Autodesk Inventor part; units mm, degrees
ref_plane "YZ Plane" through (0, 0, 0) normal (1, 0, 0) x (0, 1, 0)
ref_plane "XZ Plane" through (0, 0, 0) normal (0, 1, 0) x (-1, 0, 0)
ref_plane "XY Plane" through (0, 0, 0) normal (0, 0, 1) x (1, 0, 0)
sketch "Boceto1" plane through (0, 0, 0) normal (0, 0, 1) x (-1, 0, 0)
  line L0 (-40.5654, -5.9984) -> (-40.5654, 6.2017)
  line L1 (-40.5654, 6.2017) -> (-40.4637, 6.2017)
  line L2 (-40.4637, 6.2017) -> (-37.4137, 6.2017)
  line L3 (-37.4137, 6.2017) -> (-37.312, 6.2017)
  line L4 (-37.312, 6.2017) -> (-37.312, -5.9984)
  line L5 (-37.312, -5.9984) -> (-37.4137, -5.9984)
  line L6 (-37.4137, -5.9984) -> (-40.4637, -5.9984)
  line L7 (-40.4637, -5.9984) -> (-40.5654, -5.9984)
  line L8 (35.787, -5.9984) -> (35.6854, -5.9984)
  line L9 (35.6854, -5.9984) -> (32.6353, -5.9984)
  line L10 (32.6353, -5.9984) -> (32.5337, -5.9984)
  line L11 (32.5337, -5.9984) -> (32.5337, 6.2017)
  line L12 (32.5337, 6.2017) -> (32.6353, 6.2017)
  line L13 (32.6353, 6.2017) -> (35.6854, 6.2017)
  line L14 (35.6854, 6.2017) -> (35.787, 6.2017)
  line L15 (35.787, 6.2017) -> (35.787, -5.9984)
  line L16 (35.6854, 36.4987) -> (35.787, 36.4987)
  line L17 (35.787, 36.4987) -> (35.787, 24.2986)
  line L18 (35.787, 24.2986) -> (35.6854, 24.2986)
  line L19 (35.6854, 24.2986) -> (32.6353, 24.2986)
  line L20 (32.6353, 24.2986) -> (32.5337, 24.2986)
  line L21 (32.5337, 24.2986) -> (32.5337, 36.4987)
  line L22 (32.5337, 36.4987) -> (32.6353, 36.4987)
  line L23 (32.6353, 36.4987) -> (35.6854, 36.4987)
  line L24 (-26.0015, -48.4955) -> (-26.0015, -48.3938)
  line L25 (-26.0015, -48.3938) -> (-26.0015, -45.3438)
  line L26 (-26.0015, -45.3438) -> (-26.0015, -45.2421)
  line L27 (-26.0015, -45.2421) -> (-13.8014, -45.2421)
  line L28 (-13.8014, -45.2421) -> (-13.8014, -45.3438)
  line L29 (-13.8014, -45.3438) -> (-13.8014, -48.3938)
  line L30 (-13.8014, -48.3938) -> (-13.8014, -48.4955)
  line L31 (-13.8014, -48.4955) -> (-26.0015, -48.4955)
  line L32 (9.023, 45.4455) -> (9.023, 45.5471)
  line L33 (9.023, 45.5471) -> (9.023, 48.5971)
  line L34 (9.023, 48.5971) -> (9.023, 48.6988)
  line L35 (9.023, 48.6988) -> (21.2231, 48.6988)
  line L36 (21.2231, 48.6988) -> (21.2231, 48.5971)
  line L37 (21.2231, 48.5971) -> (21.2231, 45.5471)
  line L38 (21.2231, 45.5471) -> (21.2231, 45.4455)
  line L39 (21.2231, 45.4455) -> (9.023, 45.4455)
  line L40 (-26.0015, 45.4455) -> (-26.0015, 45.5471)
  line L41 (-26.0015, 45.5471) -> (-26.0015, 48.5971)
  line L42 (-26.0015, 48.5971) -> (-26.0015, 48.6988)
  line L43 (-26.0015, 48.6988) -> (-13.8014, 48.6988)
  line L44 (-13.8014, 48.6988) -> (-13.8014, 48.5971)
  line L45 (-13.8014, 48.5971) -> (-13.8014, 45.5471)
  line L46 (-13.8014, 45.5471) -> (-13.8014, 45.4455)
  line L47 (-13.8014, 45.4455) -> (-26.0015, 45.4455)
  line L48 (32.6353, -24.0952) -> (35.6854, -24.0952)
  line L49 (35.6854, -24.0952) -> (35.787, -24.0952)
  line L50 (35.787, -24.0952) -> (35.787, -36.2954)
  line L51 (35.787, -36.2954) -> (35.6854, -36.2954)
  line L52 (35.6854, -36.2954) -> (32.6353, -36.2954)
  line L53 (32.6353, -36.2954) -> (32.5337, -36.2954)
  line L54 (32.5337, -36.2954) -> (32.5337, -24.0952)
  line L55 (32.5337, -24.0952) -> (32.6353, -24.0952)
  line L56 (9.023, -48.4955) -> (9.023, -48.3938)
  line L57 (9.023, -48.3938) -> (9.023, -45.3438)
  line L58 (9.023, -45.3438) -> (9.023, -45.2421)
  line L59 (9.023, -45.2421) -> (21.2231, -45.2421)
  line L60 (21.2231, -45.2421) -> (21.2231, -45.3438)
  line L61 (21.2231, -45.3438) -> (21.2231, -48.3938)
  line L62 (21.2231, -48.3938) -> (21.2231, -48.4955)
  line L63 (21.2231, -48.4955) -> (9.023, -48.4955)
  line L64 (-37.4137, -36.2954) -> (-40.4637, -36.2954)
  line L65 (-40.4637, -36.2954) -> (-40.5654, -36.2954)
  line L66 (-40.5654, -36.2954) -> (-40.5654, -24.0952)
  line L67 (-40.5654, -24.0952) -> (-40.4637, -24.0952)
  line L68 (-40.4637, -24.0952) -> (-37.4137, -24.0952)
  line L69 (-37.4137, -24.0952) -> (-37.312, -24.0952)
  line L70 (-37.312, -24.0952) -> (-37.312, -36.2954)
  line L71 (-37.312, -36.2954) -> (-37.4137, -36.2954)
  line L72 (-37.312, 36.4987) -> (-37.312, 24.2986)
  line L73 (-37.312, 24.2986) -> (-37.4137, 24.2986)
  line L74 (-37.4137, 24.2986) -> (-40.4637, 24.2986)
  line L75 (-40.4637, 24.2986) -> (-40.5654, 24.2986)
  line L76 (-40.5654, 24.2986) -> (-40.5654, 36.4987)
  line L77 (-40.5654, 36.4987) -> (-40.4637, 36.4987)
  line L78 (-40.4637, 36.4987) -> (-37.4137, 36.4987)
  line L79 (-37.4137, 36.4987) -> (-37.312, 36.4987)
  line L80 (-3.05, -23.6886) -> (3.05, -23.6886)
  line L81 (3.05, -23.6886) -> (3.05, -30.8053)
  line L82 (3.05, -30.8053) -> (-3.05, -30.8053)
  line L83 (-3.05, -30.8053) -> (-3.05, -23.6886)
  circle A0 centre (-33.347, 34.9737) radius 1.4233
  circle A1 centre (28.5686, 34.9737) radius 1.4233
  circle A2 centre (0, 0) radius 7.3709
  circle A3 centre (-33.347, -32.6353) radius 1.4233
  circle A4 centre (28.5686, -32.6353) radius 1.4233
  line L84 (21.2231, 48.6988) -> (9.023, 48.6988)
  line L85 (9.023, 48.6988) -> (9.023, 45.4455)
  line L86 (9.023, 45.4455) -> (21.2231, 45.4455)
  line L87 (21.2231, 45.4455) -> (21.2231, 48.6988)
  line L88 (35.787, 36.4987) -> (32.5337, 36.4987)
  line L89 (32.5337, 36.4987) -> (32.5337, 24.2986)
  line L90 (32.5337, 24.2986) -> (35.787, 24.2986)
  line L91 (35.787, 24.2986) -> (35.787, 36.4987)
  line L92 (35.787, 6.2017) -> (32.5337, 6.2017)
  line L93 (32.5337, 6.2017) -> (32.5337, -5.9984)
  line L94 (32.5337, -5.9984) -> (35.787, -5.9984)
  line L95 (35.787, -5.9984) -> (35.787, 6.2017)
  line L96 (35.787, -24.0952) -> (32.5337, -24.0952)
  line L97 (32.5337, -24.0952) -> (32.5337, -36.2954)
  line L98 (32.5337, -36.2954) -> (35.787, -36.2954)
  line L99 (35.787, -36.2954) -> (35.787, -24.0952)
  line L100 (21.2231, -45.2421) -> (9.023, -45.2421)
  line L101 (9.023, -45.2421) -> (9.023, -48.4955)
  line L102 (9.023, -48.4955) -> (21.2231, -48.4955)
  line L103 (21.2231, -48.4955) -> (21.2231, -45.2421)
  line L104 (-13.8014, -45.2421) -> (-26.0015, -45.2421)
  line L105 (-26.0015, -45.2421) -> (-26.0015, -48.4955)
  line L106 (-26.0015, -48.4955) -> (-13.8014, -48.4955)
  line L107 (-13.8014, -48.4955) -> (-13.8014, -45.2421)
  line L108 (-37.312, -36.2954) -> (-40.5654, -36.2954)
  line L109 (-40.5654, -36.2954) -> (-40.5654, -24.0952)
  line L110 (-40.5654, -24.0952) -> (-37.312, -24.0952)
  line L111 (-37.312, -24.0952) -> (-37.312, -36.2954)
  line L112 (-37.312, -5.9984) -> (-40.5654, -5.9984)
  line L113 (-40.5654, -5.9984) -> (-40.5654, 6.2017)
  line L114 (-40.5654, 6.2017) -> (-37.312, 6.2017)
  line L115 (-37.312, 6.2017) -> (-37.312, -5.9984)
  line L116 (-37.312, 24.2986) -> (-40.5654, 24.2986)
  line L117 (-40.5654, 24.2986) -> (-40.5654, 36.4987)
  line L118 (-40.5654, 36.4987) -> (-37.312, 36.4987)
  line L119 (-37.312, 36.4987) -> (-37.312, 24.2986)
  line L120 (-26.0015, 48.6988) -> (-13.8014, 48.6988)
  line L121 (-13.8014, 48.6988) -> (-13.8014, 45.4455)
  line L122 (-13.8014, 45.4455) -> (-26.0015, 45.4455)
  line L123 (-26.0015, 45.4455) -> (-26.0015, 48.6988)
  line L124 (3.05, -23.6886) -> (-3.05, -23.6886)
  line L125 (-3.05, -23.6886) -> (-3.05, -30.8053)
  line L126 (-3.05, -30.8053) -> (3.05, -30.8053)
  line L127 (3.05, -30.8053) -> (3.05, -23.6886)
  arc A5 (40.2295, 47.3577) -> (34.4459, 53.1413) centre (34.4459, 47.3577) ccw
  line L128 (34.4459, 53.1413) -> (-39.2245, 53.1413)
  arc A6 (-39.2245, 53.1413) -> (-45.0078, 47.3579) centre (-39.2245, 47.3579) ccw
  line L129 (-45.0078, 47.3579) -> (-45.0078, -47.1423)
  arc A7 (-45.0078, -47.1423) -> (-39.2123, -52.9379) centre (-39.2123, -47.1423) ccw
  line L130 (-39.2123, -52.9379) -> (34.4339, -52.9379)
  arc A8 (34.4339, -52.9379) -> (40.2295, -47.1423) centre (34.4339, -47.1423) ccw
  line L131 (40.2295, -47.1423) -> (40.2295, 47.3577)
extrude "Extrusión1" add sketch "Boceto1" along normal blind 3
sketch "Boceto2" plane through (0, 0, 3) normal (0, 0, 1) x (1, 0, 0)
  line L0 (-34.4459, -53.1413) -> (39.2245, -53.1413)
  line L1 (39.2123, 52.9379) -> (-34.4339, 52.9379)
  line L2 (-40.2295, 47.1423) -> (-40.2295, -47.3577)
  line L3 (45.0078, -47.3579) -> (45.0078, 47.1423)
  point P0 (0, 0)
  dimension "d5" = 106.0792
  dimension "d6" = 85.2373
properties part number "tapa2"
Can you work these out from the model? Positions are in its coordinate system, mm. A direction names the side the tool comes from. Coordinates: 2 decimals unless noted, no trailing zeros. Write each loop counter-clockwise with the first axis right and the second up, starting at its lowest first coordinate (ties: lowest second). Pieces come first, ordered by that corner, then holes. Notation, with made-up numbers: M 69.5,4 L 119.5,4 A29 ccw 119.5,31 Z; hole C 18,-2 d11. An arc over 180 degrees is marked long. Write item = value, one per line. Start each with the question number.
Q1. If we section it at A-A, the plane y = 0: Write out the boundary of the cut face in (x, z), then the cut area to 3 significant figures.
Q2. If we section it at C-C, the plane x = 20.5: Write out the boundary of the cut face in (y, z), then the cut area to 3 significant figures.
Q3. If I drill on L1, parallel to Y at x = 14.5, z = 0.85; L2, parallel to X at y = 0, z = 0.7; L3, parallel to Y at x = 0, z = 0.9, over which ranges is the centre line in solid material (lowest first)? Write a range as [from, to].
Q4. If we section it at B-B, the plane x = 0: Write out the boundary of the cut face in (y, z), then the cut area to 3 significant figures.
Q5. I'm going to push a flat-ended pin straight in: pin 1 (3.5 mm diameter, centred on x = -28.57, y = -34.97, fed in from -Z). Where does the tip first touch, or does it pass through?
Q6. If we section it at D-D, the plane z = 1.75: State how many separate pieces and enclosed holes the cut face has, then the cut area to 3 significant figures.
Q7. Thinking about a two-plate mould opening in X: for faces 3 (the face through (20, 48.496, 1)), 4 (the face through (12, -1, 0)), which applies, released by +X, released by -X, zero draft, split by the parting line, or undercut?
Q8. On a 3-axis mill with a long thin cutter (end or side, diameter ignored), from which of +Z, -Z, +X, -X, +Y, -Y can I reach the whole of each face in a straight line? I mean faces 1 (the face through (-15, 48.496, 1)), 2 (the face through (3, 52.938, 1)). Say none if no direction works.
Check sheet entries:
q1.outline = M -40.23,0 L -35.79,0 L -35.79,3 L -40.23,3 Z; M -32.53,0 L -7.37,0 L -7.37,3 L -32.53,3 Z; M 7.37,0 L 37.31,0 L 37.31,3 L 7.37,3 Z; M 40.57,0 L 45.01,0 L 45.01,3 L 40.57,3 Z
q1.area = 192 mm²
q2.outline = M -53.14,0 L -48.7,0 L -48.7,3 L -53.14,3 Z; M -45.45,0 L 45.24,0 L 45.24,3 L -45.45,3 Z; M 48.5,0 L 52.94,0 L 52.94,3 L 48.5,3 Z
q2.area = 299 mm²
q3.L1 = [-53.14, -48.7], [-45.45, 45.24], [48.5, 52.94]
q3.L2 = [-40.23, -35.79], [-32.53, -7.37], [7.37, 37.31], [40.57, 45.01]
q3.L3 = [-53.14, -7.37], [7.37, 23.69], [30.81, 52.94]
q4.outline = M -53.14,0 L -7.37,0 L -7.37,3 L -53.14,3 Z; M 7.37,0 L 23.69,0 L 23.69,3 L 7.37,3 Z; M 30.81,0 L 52.94,0 L 52.94,3 L 30.81,3 Z
q4.area = 253 mm²
q5.pin_1 = 0
q6.separate_pieces = 1
q6.enclosed_holes = 16
q6.area = 8,380 mm²
q7.face_3 = undercut
q7.face_4 = zero draft
q8.face_1 = +Z, -Z
q8.face_2 = +Z, -Z, +X, -X, +Y
